from build123d import *

# Parameters (mm, degrees)
SKETCH1_W                 = 50
SKETCH1_H                 = 30
SKETCH1_R                 = 3.35
BOSS_EXTRUDE2_DEPTH       = 10
F_8_32_TAPPED_HOLE3_D     = 3.4544
F_8_32_TAPPED_HOLE3_DEPTH = 5
F_8_32_TAPPED_HOLE3_TIP   = 1.037806461
FILLET3_R                 = 2
FILLET4_R                 = 2
F_0_535_40_TAPPED_HOLE2_D = 13.2842


with BuildPart() as part:
    # Sketch1 → Boss-Extrude2 (new body)
    with BuildSketch(Plane(origin=(0, 0, 0), x_dir=(1, 0, 0), z_dir=(0, 1, 0))):
        Rectangle(SKETCH1_W, SKETCH1_H)
        with Locations((-20, 10)):
            Circle(SKETCH1_R, mode=Mode.SUBTRACT)
        with Locations((20, 10)):
            Circle(SKETCH1_R, mode=Mode.SUBTRACT)
        with Locations((-20, -10)):
            Circle(SKETCH1_R, mode=Mode.SUBTRACT)
        with Locations((20, -10)):
            Circle(SKETCH1_R, mode=Mode.SUBTRACT)
    extrude(amount=BOSS_EXTRUDE2_DEPTH)

    # #8-32 Tapped Hole3
    with Locations(Plane(origin=(0, 5, -15), x_dir=(-1, 0, 0), z_dir=(0, 0, -1))):
        with Locations((0, 0)):
            Hole(F_8_32_TAPPED_HOLE3_D / 2, depth=F_8_32_TAPPED_HOLE3_DEPTH)
            with Locations((0, 0, -(F_8_32_TAPPED_HOLE3_DEPTH + F_8_32_TAPPED_HOLE3_TIP / 2))):  # 118° drill point
                Cone(0, F_8_32_TAPPED_HOLE3_D / 2, F_8_32_TAPPED_HOLE3_TIP, mode=Mode.SUBTRACT)

    # Fillet3
    fillet3_edges = [part.edges().sort_by_distance(p)[0] for p in [
        (25, 5, 15),
        (-25, 5, -15),
        (25, 5, -15),
    ]]
    fillet(fillet3_edges, radius=FILLET3_R)

    # Fillet4
    fillet4_edges = [part.edges().sort_by_distance(p)[0] for p in [
        (-25, 5, 15),
    ]]
    fillet(fillet4_edges, radius=FILLET4_R)

    # 0.535-40 Tapped Hole2 (through all)
    with Locations(Plane.ZX.offset(10)):
        with Locations((0, 0)):
            Hole(F_0_535_40_TAPPED_HOLE2_D / 2)


solid = part.part
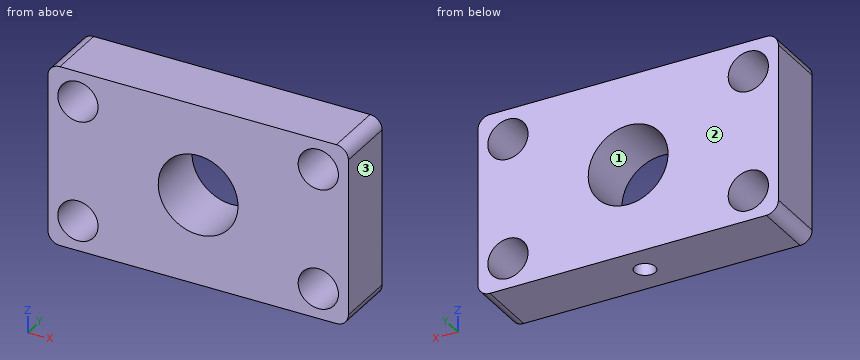
The listing builds one solid part. Answer for the finished solid, in the listing's coordinates (mm). Face numbers are marked on the shaded views. Coordinates: 2 decimals unless noted, no trailing zeros. Write each loop counter-clockwise with the first axis right and the second up, starting at its lowest first coordinate (ties: lowest second). Pieces come first, ordered by that corner, then holes. Notation, with made-up numbers: (31, 3.5) -> (62, 3.5) arc R18 ccw to (62, 24.5) -> close; hole circle Ø7 at (38.25, 9). An arc over 180 degrees is marked (long way). One line per question, with ' | ' between items.
1. Section C-C (z = -10.75) is taken. Determine the outline of the cut face in (x, y), and give its area (3 significant figures).
Verdict:
outline: (-25, 0) -> (-23.26, 0) -> (-23.26, 10) -> (-25, 10) -> close; (-16.74, 0) -> (16.74, 0) -> (16.74, 10) -> (-16.74, 10) -> close; (23.26, 0) -> (25, 0) -> (25, 10) -> (23.26, 10) -> close; hole circle Ø3.45 at (0, 5) | area: 360 mm^2
2. Section B-B (y = 8.75) is taken. Determine the outline of the cut face in (x, z), and give its area (3 significant figures).
Verdict:
outline: (-25, -13) arc R2 ccw to (-23, -15) -> (23, -15) arc R2 ccw to (25, -13) -> (25, 13) arc R2 ccw to (23, 15) -> (-23, 15) arc R2 ccw to (-25, 13) -> close; hole circle Ø6.7 at (-20, -10); hole circle Ø6.7 at (-20, 10); hole circle Ø13.28 at (0, 0); hole circle Ø6.7 at (20, -10); hole circle Ø6.7 at (20, 10) | area: 1,220 mm^2
3. Given pin 1 Ø7.5 at (x, z) = (20, 10) entering from +Y; pin 2 Ø2 at (x, y) = (0, 5) entering from -Z, each flat-ended and moving along its own axis, determine where each tip first touches the part or whether it passes through.
Verdict:
pin 1: stops at y = 10 | pin 2: stops at z = -9.56
4. For a pull along X with two mould halves and no side action, classify the marked faces 1, 2 and 3 as released by +X, released by -X, zero draft, split by the parting line, or undercut.
Verdict:
face 1: undercut | face 2: zero draft | face 3: released by +X
5. Straight lines are drawn through the part: line 1 (X direction, y = 5.25, z = 10); line 2 (Z direction, x = -20, y = 2.5); line 3 (X direction, y = 7, z = -12.5). For each, find the intervals that lie inside material, in ascending order.
Verdict:
line 1: x = -25 to -23.35, -16.65 to 16.65, 23.35 to 25 | line 2: z = -15 to -13.35, -6.65 to 6.65, 13.35 to 15 | line 3: x = -25 to -22.23, -17.77 to 17.77, 22.23 to 25
6. Section A-A (z = 0) is taken. Determine the outline of the cut face in (x, y).
Verdict:
outline: (-25, 0) -> (-6.64, 0) -> (-6.64, 10) -> (-25, 10) -> close; (6.64, 0) -> (25, 0) -> (25, 10) -> (6.64, 10) -> close
7. Section D-D (x = -3) is taken. Determine the outline of the cut face in (y, z), and give its area (3 significant figures).
Verdict:
outline: (0, -15) -> (10, -15) -> (10, -5.93) -> (0, -5.93) -> close; (0, 5.93) -> (10, 5.93) -> (10, 15) -> (0, 15) -> close | area: 181 mm^2
